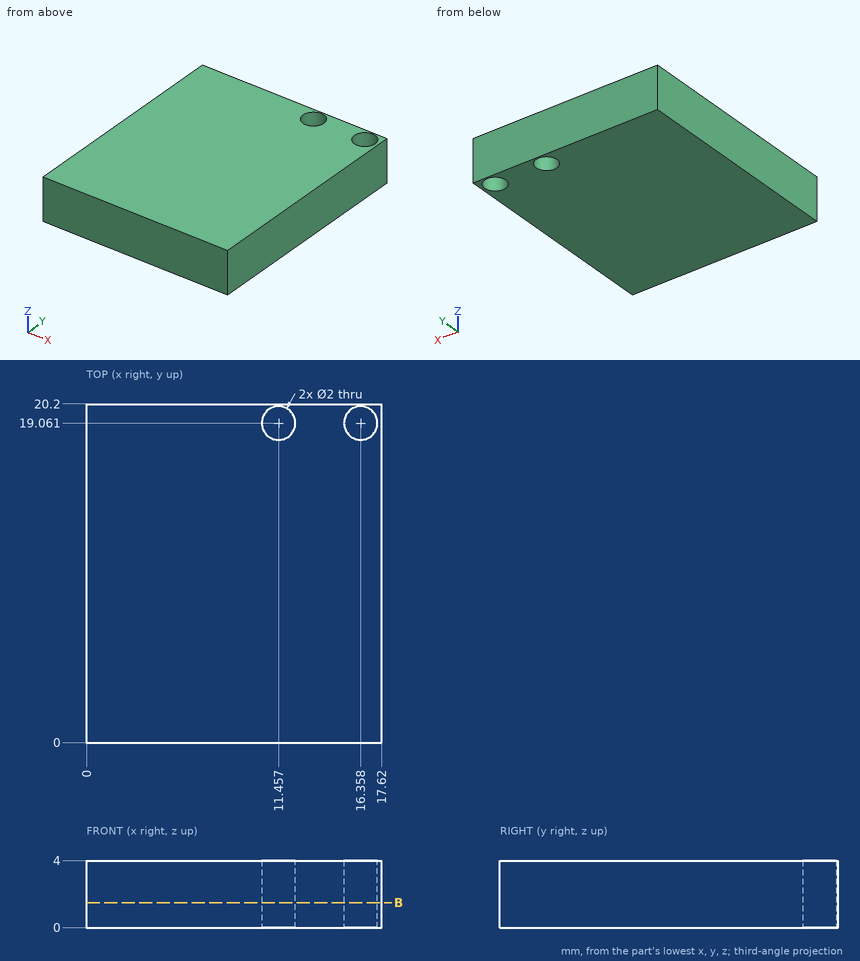
Could you check a few things on this drawing? It's one solid part, dimensions in mm from its lowest x, y, z. Give positions to 0.01 mm unless a question says otherwise; leave off trailing zeros. Order: outer loops, then holes, each group sorted by start corner. A loop starts at its lowest first (then second) coordinate and runs counter-clockwise, first axis right, second up. Notation, with made-up numbers: (-35.5, -7.5) - (-27.5, -7.5) arc R19 cw to (-27.5, 14.5) - close; hole circle Ø10 at (46.5, -3). An arc over 180 degrees is marked (long way). One line per item, written item: value. Start each with the question number.
1. For P1, Ø2.5, axis at x = 16.36, y = 19.06, coming from the +Z side, with a flat end and sliding along its axis, tell me the tip position at first contact or that it passes through.
2. Imagine slicing it at B-B on z = 1.5. List the corners of the cut face in (x, y) for me, plus the area to 3 significant figures.
3. If I drill on probe 1 along X at (y, z) = (18.25, 0.55) (1 decimal); probe 2 along Y at (x, z) = (16, 2.05) (1 decimal), over which ranges is the centre line in solid material (lowest first)?
Values:
1. P1: z = 4
2. outline: (0, 0) - (17.62, 0) - (17.62, 20.2) - (0, 20.2) - close; hole circle Ø2 at (11.46, 19.06); hole circle Ø2 at (16.36, 19.06)
2. area: 350 mm²
3. probe 1: 0 to 10.9, 12 to 15.8, 16.9 to 17.6
3. probe 2: 0 to 18.1, 20 to 20.2
